from build123d import *

# Parameters (mm, degrees)
SKETCH2_W          = 14
SKETCH2_H          = 10
CUT_EXTRUDE1_DEPTH = 73
SKETCH3_R          = 8
CUT_EXTRUDE2_DEPTH = 217
CIRPATTERN1_COUNT  = 4


with BuildPart() as part:
    # Sketch1 → Revolve1 (revolve)
    with BuildSketch(Plane(origin=(0, 0, 0), x_dir=(0, 0, -1), z_dir=(1, 0, 0)), mode=Mode.PRIVATE) as revolve1_sk:
        Polygon((-44, 104), (0, 104), (0, 48), (3, 48), (3, 25), (-54, 25), (-54, 48), (-24, 48), (-24, 98), (-44, 98), align=None)
    revolve(revolve1_sk.sketch.rotate(Axis((0, 0, 52.496471852), (0, 0, -1)), 90), axis=Axis((0, 0, 52.496471852), (0, 0, -1)))

    # Sketch2 → Cut-Extrude1 (cut, symmetric)
    with BuildSketch(Plane.XY):
        with Locations((0, 25)):
            Rectangle(SKETCH2_W, SKETCH2_H)
    extrude(amount=CUT_EXTRUDE1_DEPTH, both=True, mode=Mode.SUBTRACT)

    # Sketch3 → Cut-Extrude2 (cut)
    with BuildSketch(Plane.XY):
        with Locations(Location((0, 78.704447468, 0), (0, 0, 180))):
            Circle(SKETCH3_R)
    cut_extrude2 = extrude(amount=CUT_EXTRUDE2_DEPTH, mode=Mode.SUBTRACT)

    # CirPattern1: Cut-Extrude2 ×4 about axis
    cirpattern1_axis = Axis((0, 0, 0), (0, 0, 1))
    for i in range(1, CIRPATTERN1_COUNT):
        add(cut_extrude2.rotate(cirpattern1_axis, i * 360 / CIRPATTERN1_COUNT), mode=Mode.SUBTRACT)


solid = part.part
Work out the finished part from the listing and answer in its coordinate system (mm). A direction names the side the tool comes from. Round coordinates to 2 decimals unless told otherwise and drop trailing zeros. Loops run counter-clockwise (first coordinate to the right, second up) from the corner with the lowest first, then second, coordinate; pieces in that order, holes last. Notation, with made-up numbers: M 61,50.5 L 116,50.5 A23 ccw 116,64.5 Z; hole C 27,46 d5. An arc over 180 degrees is marked long. One line per question, with ' | ' between items. Start each with the question number.
(1) A cutting plane is placed at C-C on x = 0. Write down the section's boundary in (y, z).
(2) Find the intervals of material crossed by line 1 (Y direction, x = 0, z = 37); line 2 (Y direction, x = 0, z = 12.75); line 3 (X direction, y = -9, z = 29), in increasing order.
(3) A cutting plane is placed at A-A on z = 36.5. Write down the section's boundary in (x, y), plus the area to 3 significant figures.
(4) A cutting plane is placed at B-B on y = 0. Write down the section's boundary in (x, z).
(5) Flat-ended cylindrical pins translate along their axes: pin 1 Ø6.5 at (y, z) = (25.5, 19.5) entering from -X; pin 2 Ø3 at (x, z) = (-47.5, 4) entering from -Y; pin 3 Ø5 at (y, z) = (26.5, 19.5) entering from +X. Find the tip coordinate at first contact, or state that the pin passes through.
(6) A cutting plane is placed at D-D on y = -83.5. Write down the section's boundary in (x, z), plus the area to 3 significant figures.
(7) For a pull along Y with two mould halves and no side action, classify faces 1 (the face through (45.783, -14.418, -1.521)), 2 (the face through (1, -24.98, 25.9)), 3 (the face through (-21, 21, 54)) as released by +Y, released by -Y, zero draft, split by the parting line, or undercut.
(8) A tool of negligible diameter and unlimited length cuts with its end or side. For faces 4 (the face through (45, 22, 0)), 5 (the face through (21, 21, -3)), 6 (the face through (45.783, -14.418, 38.79)), 7 (the face through (-7, 27, 26)), from which of +Z, -Z, +X, -X, +Y, -Y can it reach the whole face along a straight path? Write none if from no direction.
Geometry check:
1) outline: M -104,0 L -86.7,0 L -86.7,24 L -98,24 L -98,44 L -104,44 Z; M -70.7,0 L -48,0 L -48,-3 L -25,-3 L -25,54 L -48,54 L -48,24 L -70.7,24 Z; M 30,-3 L 48,-3 L 48,0 L 70.7,0 L 70.7,24 L 48,24 L 48,54 L 30,54 Z; M 86.7,0 L 104,0 L 104,44 L 98,44 L 98,24 L 86.7,24 Z
2) line 1: y = -104 to -98, -48 to -25, 30 to 48, 98 to 104 | line 2: y = -104 to -86.7, -70.7 to -25, 30 to 70.7, 86.7 to 104 | line 3: x = -103.61 to -97.59, -47.15 to -23.32, 23.32 to 47.15, 97.59 to 103.61
3) outline: C 0,0 d208; C 0,0 d96; hole C 0,0 d196; hole M -7,24 A25 ccw long 7,24 L 7,30 L -7,30 Z | area: 9,010 mm²
4) outline: M -104,0 L -86.7,0 L -86.7,24 L -98,24 L -98,44 L -104,44 Z; M -70.7,0 L -48,0 L -48,-3 L -25,-3 L -25,54 L -48,54 L -48,24 L -70.7,24 Z; M 25,-3 L 48,-3 L 48,0 L 70.7,0 L 70.7,24 L 48,24 L 48,54 L 25,54 Z; M 86.7,0 L 104,0 L 104,44 L 98,44 L 98,24 L 86.7,24 Z
5) pin 1: stops at x = -101.59 | pin 2: stops at y = -93.27 | pin 3: stops at x = 101.19
6) outline: M -62,0 L -6.4,0 L -6.4,24 L -51.3,24 L -51.3,44 L -62,44 Z; M 6.4,0 L 62,0 L 62,44 L 51.3,44 L 51.3,24 L 6.4,24 Z | area: 3,100 mm²
7) face 1: split by the parting line | face 2: undercut | face 3: zero draft
8) face 4: -Z | face 5: -Z, +X, -X, +Y, -Y | face 6: +Z | face 7: +Z, -Z
